Answer from the drawing. Dimensions are ordinates in mm from the lowest x, y and z of the part. A direction names the side the tool comes from. Round coordinates to 2 decimals unless told otherwise and drop trailing zeros. Write each loop counter-clockwise with the first axis right and the second up, starting at its lowest first coordinate (ties: lowest second). Pieces come first, ordered by that corner, then holes. Notation, with made-up numbers: (-26, 51.5) -> (27, 51.5) arc R21 cw to (27, 89.5) -> close; hole circle Ø4 at (-39.75, -37.5). An arc over 180 degrees is marked (long way). Return JSON: item names as keys, results as strings. Group by question number.
(1) Straight lines are drawn through the part: line 1 (Y direction, x = 30, z = 15.5); line 2 (Y direction, x = 45, z = 29); line 3 (Y direction, x = 3, z = 10.5). For each, find the intervals that lie inside material, in ascending order.
(2) The mould has two halves that part along X. Classify the marked faces 4, 5, 6 and 7: released by +X, released by -X, zero draft, split by the parting line, or undercut.
(3) A cutting plane is placed at A-A on x = 25.5. Give the vertices of the cut face in (y, z).
(4) A cutting plane is placed at C-C on y = 49.5. Give the vertices of the cut face in (x, z), then the cut area to 3 significant figures.
(5) Given pin 1 (3 mm diameter, centred on y = 31, z = 21.5, fed in from -X); pin 2 (2 mm diameter, centred on x = 25.5, z = 27, fed in from +Y); pin 3 (3.5 mm diameter, centred on y = 75, z = 22.5, fed in from -X); pin 4 (15 mm diameter, centred on x = 30.5, z = 26.5, fed in from -Y), each flat-ended and moving along its own axis, determine where each tip first touches the part or whether it passes through.
(6) A cutting plane is placed at D-D on x = 67.5. Give the vertices of the cut face in (y, z).
(7) For the marked faces 1, 2 and 3, determine the directions among +Z, -Z, +X, -X, +Y, -Y from which every point of the face is accessible in a straight line to the end or side of a thin tool.
(8) A cutting plane is placed at B-B on z = 8.5. Give the vertices of the cut face in (x, y).
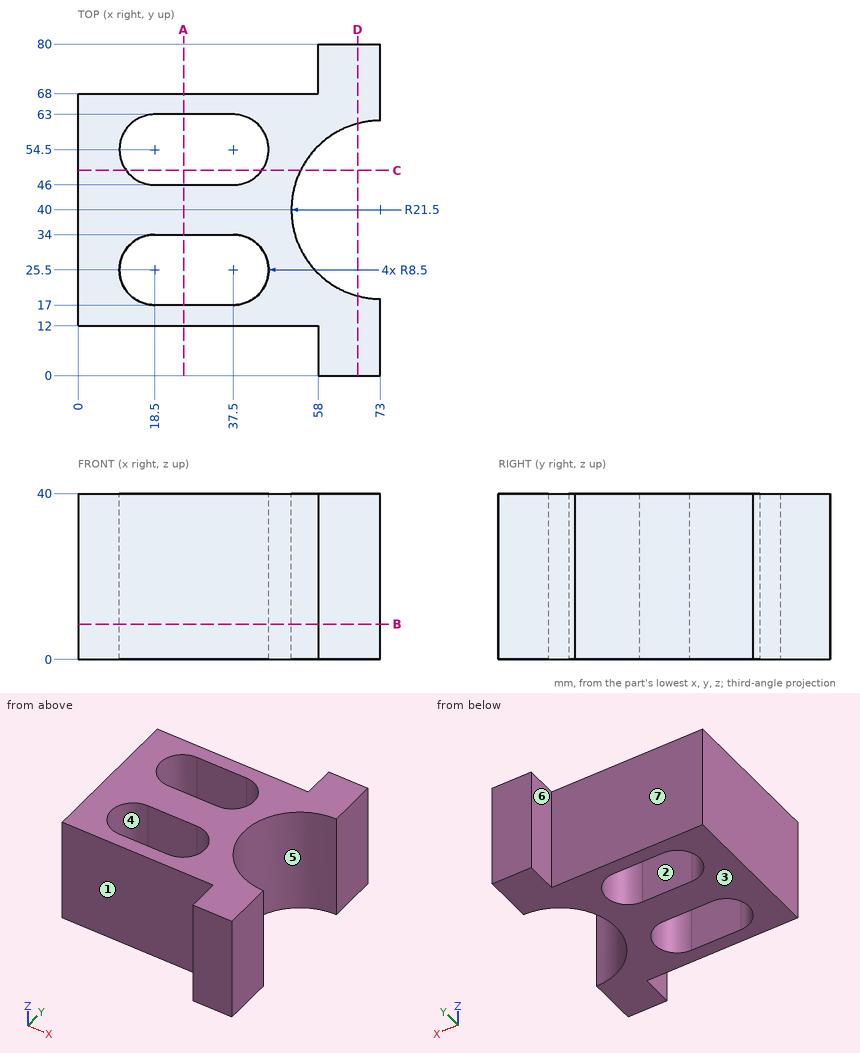
Checks:
{
 "1": {"line 1": "y = 12 to 17, 34 to 46, 63 to 68", "line 2": "y = 12 to 21.5, 29.5 to 50.5, 58.5 to 68", "line 3": "y = 12 to 68"},
 "2": {"face 4": "undercut", "face 5": "released by +X", "face 6": "released by -X", "face 7": "zero draft"},
 "3": {"outline": "(12, 0) -> (17, 0) -> (17, 40) -> (12, 40) -> close; (34, 0) -> (46, 0) -> (46, 40) -> (34, 40) -> close; (63, 0) -> (68, 0) -> (68, 40) -> (63, 40) -> close"},
 "4": {"outline": "(0, 0) -> (11.63, 0) -> (11.63, 40) -> (0, 40) -> close; (44.37, 0) -> (53.71, 0) -> (53.71, 40) -> (44.37, 40) -> close", "area": "839 mm^2"},
 "5": {"pin 1": "stops at x = 0", "pin 2": "stops at y = 68", "pin 3": "stops at x = 58", "pin 4": "stops at y = 12"},
 "6": {"outline": "(0, 0) -> (19.22, 0) -> (19.22, 40) -> (0, 40) -> close; (60.78, 0) -> (80, 0) -> (80, 40) -> (60.78, 40) -> close"},
 "7": {"face 1": "+Z, -Z, -X, -Y", "face 2": "+Z, -Z", "face 3": "-Z, +X, -X, +Y, -Y"},
 "8": {"outline": "(0, 12) -> (58, 12) -> (58, 0) -> (73, 0) -> (73, 18.5) arc R21.5 cw to (73, 61.5) -> (73, 80) -> (58, 80) -> (58, 68) -> (0, 68) -> close; hole (18.5, 17) -> (37.5, 17) arc R8.5 ccw to (37.5, 34) -> (18.5, 34) arc R8.5 ccw to start; hole (18.5, 46) -> (37.5, 46) arc R8.5 ccw to (37.5, 63) -> (18.5, 63) arc R8.5 ccw to start"}
}
